For this review, take the finished solid that the model builds, in its own axes (mm). Round coordinates to 2 decimals unless told otherwise and drop trailing zeros. Write each loop counter-clockwise with the first axis right and the second up, starting at its lowest first coordinate (ties: lowest second). Pieces come first, ordered by that corner, then holes. Notation, with made-up numbers: M 75.25,59 L 117.25,59 A17 cw 117.25,73 Z; hole C 55,73 d2. An arc over 180 degrees is marked long. One line per question, with ' | ' between items.
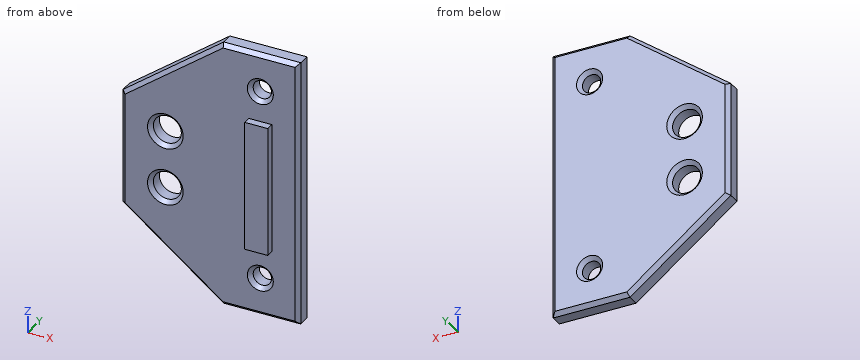
```python
from build123d import *

# Parameters (mm, degrees)
ESBO_O1_R                = 3.625
ESBO_O1_R_2              = 2.375
RESSALTO_EXTRUS_O1_DEPTH = 5
CHANFRO2_SIZE            = 1
ESBO_O2_W                = 6
ESBO_O2_H                = 34
RESSALTO_EXTRUS_O2_DEPTH = 2


with BuildPart() as part:
    # Esboço1 → Ressalto-extrusão1 (new body)
    with BuildSketch(Plane(origin=(0, 0, 0), x_dir=(1, 0, 0), z_dir=(0, 1, 0))):
        Polygon((-23.080933084, -15), (3.080933084, -15), (3.080933084, -35), (23.080933084, -35), (23.080933084, -15), (23.080933084, 15), (23.080933084, 35), (3.080933084, 35), (3.080933084, 15), (-23.080933084, 15), align=None)
        with Locations((-11.580933084, -7.5)):
            Circle(ESBO_O1_R, mode=Mode.SUBTRACT)
        with Locations((-11.580933084, 7.5)):
            Circle(ESBO_O1_R, mode=Mode.SUBTRACT)
        with Locations((13.080933084, -25)):
            Circle(ESBO_O1_R_2, mode=Mode.SUBTRACT)
        with Locations((13.080933084, 25)):
            Circle(ESBO_O1_R_2, mode=Mode.SUBTRACT)
        Polygon((-23.080933084, 15), (3.080933084, 15), (3.080933084, 35), align=None)
        Polygon((3.080933084, -15), (3.080933084, -35), (-23.080933084, -15), align=None)
    extrude(amount=RESSALTO_EXTRUS_O1_DEPTH)

    # Chanfro2
    chanfro2_edges = [part.edges().sort_by_distance(p)[0] for p in [
        (10.705933084, 0, -25),
        (10.705933084, 0, 25),
        (-10, 5, -25),
        (-15.205933084, 0, -7.5),
        (-15.205933084, 0, 7.5),
        (23.080933084, 0, 0),
        (13.080933084, 0, 35),
        (-10, 0, 25),
        (-23.080933084, 0, 0),
        (-10, 0, -25),
        (-23.080933084, 5, 0),
        (13.080933084, 0, -35),
        (-10, 5, 25),
        (13.080933084, 5, 35),
        (23.080933084, 5, 0),
        (-15.205933084, 5, 7.5),
        (-15.205933084, 5, -7.5),
        (10.705933084, 5, 25),
        (10.705933084, 5, -25),
        (13.080933084, 5, -35),
    ]]
    chamfer(chanfro2_edges, length=CHANFRO2_SIZE)

    # Esboço2 → Ressalto-extrusão2 (add)
    with BuildSketch(Plane.XZ):
        with Locations((13.080933084, 0)):
            Rectangle(ESBO_O2_W, ESBO_O2_H)
    extrude(amount=RESSALTO_EXTRUS_O2_DEPTH)


solid = part.part
```
Item 1: Take a section at B-B (x = 18). Write out the cut boundary in (y, z).
Results:
outline: M 0,-34 L 1,-35 L 4,-35 L 5,-34 L 5,34 L 4,35 L 1,35 L 0,34 Z
Item 2: Insertion check: pin 1 Ø0.6 at (x, y) = (13, -0.5) entering from -Z; pin 2 Ø5.5 at (x, z) = (13.08, 25) entering from -Y; pin 3 Ø2 at (y, z) = (-1.5, -8) entering from +X; pin 4 Ø6.5 at (x, z) = (-11.58, 7.5) entering from +Y. Each pin has a flat end and moves straight along its axis. Give the tip position at first contact, or say it passes through.
Results:
pin 1: z = -17 | pin 2: y = 0.62 | pin 3: x = 16.08 | pin 4: through
Item 3: Take a section at A-A (z = -7.5). Write out the cut boundary in (x, y), then the cut area to 3 significant figures.
Results:
outline: M -23.08,1 L -22.08,0 L -16.21,0 L -15.21,1 L -15.21,4 L -16.21,5 L -22.08,5 L -23.08,4 Z; M -7.96,1 L -6.96,0 L 10.08,0 L 10.08,-2 L 16.08,-2 L 16.08,0 L 22.08,0 L 23.08,1 L 23.08,4 L 22.08,5 L -6.96,5 L -7.96,4 Z | area: 203 mm2
Item 4: Take a section at C-C (y = -1.25). Write out the cut boundary in (x, z), then the cut area to 3 significant figures.
Results:
outline: M 10.08,-17 L 16.08,-17 L 16.08,17 L 10.08,17 Z | area: 204 mm2
Item 5: Take a section at D-D (z = -25). Write out the cut boundary in (x, y).
Results:
outline: M -10,1 L -8.35,0 L 9.71,0 L 10.71,1 L 10.71,4 L 9.71,5 L -8.35,5 L -10,4 Z; M 15.46,1 L 16.46,0 L 22.08,0 L 23.08,1 L 23.08,4 L 22.08,5 L 16.46,5 L 15.46,4 Z
Item 6: To check wall thickness, follow line 1 along Z through (x, y) = (-12.5, 2); line 2 along X through (y, z) = (3.35, 7.5); line 3 along Y through (x, z) = (9.5, -15.5). State the ranges of each line that lie inside material, in increasing order. Write a range as from..to.
Results:
line 1: -23.09..-11.01, -3.99..3.99, 11.01..23.09 | line 2: -23.08..-15.21, -7.96..23.08 | line 3: 0..5
